from build123d import *

# Parameters (mm, degrees)
SKETCH_2_R          = 1.5
EXTRUDE_2_DEPTH     = 5
EXTRUDE_2_2_DEPTH   = 5
EXTRUDE_2_3_DEPTH   = 5
EXTRUDE_5_DEPTH     = 2
EXTRUDE_6_DEPTH     = 2
EXTRUDE_7_DEPTH     = 5
SKETCH_11_R         = 1.25
EXTRUDE_8_DEPTH     = 5
CHAMFER_1_SIZE      = 4
SKETCH_12_R         = 2
CUT_EXTRUDE_1_DEPTH = 2


with BuildPart() as part:
    # Sketch 2 → Extrude 2 (new body)
    with BuildSketch(Plane(origin=(0, 0, 0), x_dir=(1, 0, 0), z_dir=(0, 1, 0))):
        Polygon((7.2, 29.088730163), (7.2, 34.911269837), (3.911269837, 38.2), (-3.911269837, 38.2), (-7.2, 34.911269837), (-7.2, 29.088730163), (-3.911269837, 25.8), (3.911269837, 25.8), align=None)
        with Locations(Location((0, 32, 0), (0, 0, 270))):
            Circle(SKETCH_2_R, mode=Mode.SUBTRACT)
    extrude(amount=-EXTRUDE_2_DEPTH)



with BuildPart() as body_2:
    # Sketch 2 → Extrude 2 2 (new body)
    with BuildSketch(Plane(origin=(0, 0, 0), x_dir=(1, 0, 0), z_dir=(0, 1, 0))):
        Polygon((20, -24), (20, -33), (20, -34.2), (21.911269837, -34.2), (33.2, -22.911269837), (33.2, -19), (25, -19), align=None)
        with Locations(Location((25, -24, 0), (0, 0, 270))):
            Circle(SKETCH_2_R, mode=Mode.SUBTRACT)
    extrude(amount=-EXTRUDE_2_2_DEPTH)

    # Sketch 5 → Extrude 6 (add)
    with BuildSketch(Plane(origin=(0, 0, 0), x_dir=(1, 0, 0), z_dir=(0, 1, 0))):
        Polygon((31.2, -19), (33.2, -19), (33.2, -22.911269837), (21.911269837, -34.2), (20, -34.2), (20, -33.282842712), (31.2, -22.082842712), align=None)
    extrude(amount=EXTRUDE_6_DEPTH)


with BuildPart() as body_3:
    # Sketch 2 → Extrude 2 3 (new body)
    with BuildSketch(Plane(origin=(0, 0, 0), x_dir=(1, 0, 0), z_dir=(0, 1, 0))):
        Polygon((-20, -34.2), (-20, -24), (-23, -21), (-34.2, -21), (-34.2, -24.911269837), (-24.911269837, -34.2), align=None)
        with Locations(Location((-25, -24, 0), (0, 0, 270))):
            Circle(SKETCH_2_R, mode=Mode.SUBTRACT)
    extrude(amount=-EXTRUDE_2_3_DEPTH)


with BuildPart() as part_1:
    add(part.part)

    add(body_3.part)  # Extrude 5 merges body 3
    # Sketch 3 → Extrude 5 (add)
    with BuildSketch(Plane(origin=(0, 0, 0), x_dir=(1, 0, 0), z_dir=(0, 1, 0))):
        Polygon((7.2, 30.2), (7.2, 34.911269837), (3.911269837, 38.2), (-3.911269837, 38.2), (-7.2, 34.911269837), (-7.2, 30.2), (-6.082842712, 30.2), (-5.2, 31.082842712), (-5.2, 34.082842712), (-3.082842712, 36.2), (3.082842712, 36.2), (5.2, 34.082842712), (5.2, 31.082842712), (6.082842712, 30.2), align=None)
        Polygon((-24.911269837, -34.2), (-20, -34.2), (-20, -32.2), (-24.082842712, -32.2), (-32.2, -24.082842712), (-32.2, -21), (-34.2, -21), (-34.2, -24.911269837), align=None)
    extrude(amount=EXTRUDE_5_DEPTH)


    add(body_2.part)  # Extrude 7 merges body 2
    # Sketch 6 → Extrude 7 (add)
    with BuildSketch(Plane.XZ.offset(5)):
        Polygon((-7.2, -34.911269837), (-3.911269837, -38.2), (3.911269837, -38.2), (7.2, -34.911269837), (9.022539674, -33.088730163), (19.022539674, -33.088730163), (33.2, -18.911269837), (33.2, 19), (33.2, 22.911269837), (21.911269837, 34.2), (19.111269837, 37), (13, 37), (-8, 37), (-22.111269837, 37), (-24.911269837, 34.2), (-34.2, 24.911269837), (-34.2, 21), (-34.2, -24.088730163), (-25.2, -33.088730163), (-9.022539674, -33.088730163), align=None)
        Polygon((7.2, -29.088730163), (3.911269837, -25.8), (-3.911269837, -25.8), (-7.2, -29.088730163), (-23.543145751, -29.088730163), (-31.2, -21.431875913), (-31.2, 19.425988463), (-29.625988463, 21), (-23, 21), (-20, 24), (-20, 30.625988463), (-17.625988463, 33), (14.625988463, 33), (20, 27.625988463), (20, 24), (25, 19), (29.2, 14.8), (29.2, -17.254415588), (17.365685425, -29.088730163), align=None, mode=Mode.SUBTRACT)
    extrude(amount=EXTRUDE_7_DEPTH)

    # Sketch 11 → Extrude 8 (add)
    # profile 1 of 3: a face of its own
    with BuildSketch(Plane(origin=(0, -5, 0), x_dir=(1, 0, 0), z_dir=(0, 1, 0))):
        with BuildLine():
            Line((41.053919682, 12), (33.2, 12))
            Line((33.2, 12), (33.2, -12))
            Line((33.2, -12), (41.053919682, -12))
            Line((41.053919682, -12), (43.053919682, -10))
            ThreePointArc((43.053919682, -10), (44.2, 0), (43.053919682, 10))
            Line((43.053919682, 10), (41.053919682, 12))
        make_face()
        with Locations(Location((39, 8, 0), (0, 0, 270))):
            Circle(SKETCH_11_R, mode=Mode.SUBTRACT)
        with Locations(Location((39, -8, 0), (0, 0, 270))):
            Circle(SKETCH_11_R, mode=Mode.SUBTRACT)
    # profile 2 of 3: a face of its own
    with BuildSketch(Plane(origin=(0, -5, 0), x_dir=(1, 0, 0), z_dir=(0, 1, 0))):
        with BuildLine():
            Line((-41.053919682, 12), (-34.2, 12))
            Line((-34.2, 12), (-34.2, -12))
            Line((-34.2, -12), (-41.053919682, -12))
            Line((-41.053919682, -12), (-43.053919682, -10))
            ThreePointArc((-43.053919682, -10), (-44.2, 0), (-43.053919682, 10))
            Line((-43.053919682, 10), (-41.053919682, 12))
        make_face()
        with Locations(Location((-39, 8, 0), (0, 0, 90))):
            Circle(SKETCH_11_R, mode=Mode.SUBTRACT)
        with Locations(Location((-39, -8, 0), (0, 0, 90))):
            Circle(SKETCH_11_R, mode=Mode.SUBTRACT)
    # profile 3 of 3: a face of its own
    with BuildSketch(Plane(origin=(0, -5, 0), x_dir=(1, 0, 0), z_dir=(0, 1, 0))):
        Polygon((-12, -42.44), (12, -42.44), (17.44, -37), (-17.44, -37), align=None)
        with Locations(Location((8, -39.23, 0), (0, 0, 270))):
            Circle(SKETCH_11_R, mode=Mode.SUBTRACT)
        with Locations(Location((-8, -39.23, 0), (0, 0, 90))):
            Circle(SKETCH_11_R, mode=Mode.SUBTRACT)
    extrude(amount=-EXTRUDE_8_DEPTH)

    # Chamfer 1
    chamfer_1_edges = [part_1.edges().sort_by_distance(p)[0] for p in [
        (33.2, -7.5, 12),
        (33.2, -7.5, -12),
        (-34.2, -7.5, -12),
        (-34.2, -7.5, 12),
    ]]
    chamfer(chamfer_1_edges, length=CHAMFER_1_SIZE)

    # Sketch 12 → Cut-Extrude 1 (cut)
    with BuildSketch(Plane(origin=(0, -5, 0), x_dir=(1, 0, 0), z_dir=(0, 1, 0))):
        with Locations(Location((-39, 8, 0), (0, 0, 270))):
            Circle(SKETCH_12_R)
        with Locations(Location((-39, -8, 0), (0, 0, 270))):
            Circle(SKETCH_12_R)
        with Locations(Location((39, 8, 0), (0, 0, 270))):
            Circle(SKETCH_12_R)
        with Locations(Location((39, -8, 0), (0, 0, 270))):
            Circle(SKETCH_12_R)
        with Locations(Location((8, -39.23, 0), (0, 0, 270))):
            Circle(SKETCH_12_R)
        with Locations(Location((-8, -39.23, 0), (0, 0, 270))):
            Circle(SKETCH_12_R)
    extrude(amount=-CUT_EXTRUDE_1_DEPTH, mode=Mode.SUBTRACT)


solid = part_1.part
Work out the finished part from the listing and answer in its coordinate system (mm). A direction names the side the tool comes from. Give positions to 0.01 mm unless a question says otherwise; leave off trailing zeros. Order: outer loops, then holes, each group sorted by start corner. A loop starts at its lowest first (then second) coordinate and runs counter-clockwise, first axis right, second up. Notation, with made-up numbers: M 66,75 L 85,75 A33 ccw 85,110 Z; hole C 12,19.5 d9. An arc over 180 degrees is marked long. Return JSON: item names as keys, results as strings.
Q1. Which of the six approach directions +Z, -Z, +X, -X, +Y, -Y give full straight-line access (tool end or side, diameter ignored) to faces 1 (the face through (5.2, 1, -33)), 2 (the face through (-34.2, -7, -20)), 3 (the face through (-9, -7, 38)), 4 (the face through (39, -7, -12))?
Answer below:
{"face 1": "+Z, +Y", "face 2": "-Z, -X, +Y, -Y", "face 3": "+Y", "face 4": "-Z, +X, +Y, -Y"}
Q2. Find section A-A, the plane y = -3.5. Write down the section's boundary in (x, z).
Answer below:
{"outline": "M -34.2,21 L -23,21 L -20,24 L -20,34.2 L -24.91,34.2 L -34.2,24.91 Z; M -7.2,-34.91 L -3.91,-38.2 L 3.91,-38.2 L 7.2,-34.91 L 7.2,-29.09 L 3.91,-25.8 L -3.91,-25.8 L -7.2,-29.09 Z; M 20,24 L 25,19 L 33.2,19 L 33.2,22.91 L 21.91,34.2 L 20,34.2 Z; hole C -25,24 d3; hole C 0,-32 d3; hole C 25,24 d3"}
Q3. Each of these flat-tipped pins is pushed along its axis until it touches: pin 1 (5 mm diameter, centred on x = 0, z = -32, fed in from +Y); pin 2 (1.5 mm diameter, centred on x = 39, z = 8, fed in from +Y); pin 3 (2.5 mm diameter, centred on y = -7, z = -18.5, fed in from -X); pin 4 (4 mm diameter, centred on y = -8, z = -28, fed in from +X). Where does it stop, or does it pass through?
Answer below:
{"pin 1": "stops at y = 0", "pin 2": "passes through", "pin 3": "stops at x = -34.2", "pin 4": "stops at x = 26.11"}
Q4. Find section B-B, the plane x = 13.5. Write down the section's boundary in (y, z).
Answer below:
{"outline": "M -10,-33.09 L -5,-33.09 L -5,-29.09 L -10,-29.09 Z; M -10,33 L -5,33 L -5,40.94 L -10,40.94 Z"}
Q5. The mould has two halves that part along X. Classify faces 5 (the face through (7.2, -2, -32)), 6 (the face through (0, -5, -25.8)), 7 (the face through (-28, 2, 29)), 8 (the face through (-42.068, -7.465, -10.986)): pulls with the +X half, pulls with the -X half, needs draft (parallel to the pull), parting line crosses it, or undercut.
Answer below:
{"face 5": "pulls with the +X half", "face 6": "undercut", "face 7": "needs draft", "face 8": "pulls with the -X half"}
Q6. Find section D-D, the plane z = -8. Write down the section's boundary in (x, y).
Answer below:
{"outline": "M -43.47,-10 L -40.25,-10 L -40.25,-7 L -41,-7 L -41,-5 L -43.47,-5 Z; M -37.75,-10 L -31.2,-10 L -31.2,-5 L -37,-5 L -37,-7 L -37.75,-7 Z; M 29.2,-10 L 37.75,-10 L 37.75,-7 L 37,-7 L 37,-5 L 29.2,-5 Z; M 40.25,-10 L 43.47,-10 L 43.47,-5 L 41,-5 L 41,-7 L 40.25,-7 Z"}
Q7. Find section C-C, the plane z = 39.23. Write down the section's boundary in (x, y), and give its area (3 significant figures).
Answer below:
{"outline": "M -15.21,-10 L -9.25,-10 L -9.25,-7 L -10,-7 L -10,-5 L -15.21,-5 Z; M -6.75,-10 L 6.75,-10 L 6.75,-7 L 6,-7 L 6,-5 L -6,-5 L -6,-7 L -6.75,-7 Z; M 9.25,-10 L 15.21,-10 L 15.21,-5 L 10,-5 L 10,-7 L 9.25,-7 Z", "area": "121 mm^2"}
Q8. Find the intervals of material crossed by line 1 along Z through (x, y) = (-21.5, -9); line 2 along X through (y, z) = (-8.75, 39.5); line 3 along X through (y, z) = (-5.95, 39.23), in increasing order. Write a range as [from, to].
Answer below:
{"line 1": "z = [-33.09, -29.09], [22.5, 37]", "line 2": "x = [-14.94, -9.22], [-6.78, 6.78], [9.22, 14.94]", "line 3": "x = [-15.21, -10], [-6, 6], [10, 15.21]"}
